Verification items for the finished model (mm, model axes). A direction names the side the tool comes from. Round coordinates to 2 decimals unless told otherwise and drop trailing zeros. Loops run counter-clockwise (first coordinate to the right, second up) from the corner with the lowest first, then second, coordinate; pieces in that order, holes last. Notation, with made-up numbers: M 27.25,88.5 L 39.25,88.5 A28 cw 39.25,115.5 Z; hole C 56,-10 d9. An arc over 180 degrees is marked long. Write item = value, one per line. Start each with the question number.
from build123d import *

# Parameters (mm, degrees)
EXTRUDE_THIN1_DEPTH = 34.154055886
SKETCH5_R           = 1.15
SKETCH5_W           = 12.978284002
SKETCH5_H           = 24
CUT_EXTRUDE7_DEPTH  = 8
SKETCH6_W           = 17.6
SKETCH6_H           = 13.993236592
SKETCH6_H_2         = 12.157086016
CUT_EXTRUDE8_DEPTH  = 29
SKETCH7_R           = 1.45
CUT_EXTRUDE9_DEPTH  = 33
SKETCH8_W           = 25.782103653
SKETCH8_H           = 13.229301
CUT_EXTRUDE10_DEPTH = 16


with BuildPart() as part:
    # Sketch1 → Extrude-Thin1 (new body)
    with BuildSketch(Plane.XY):
        Polygon((17.6, 0), (0, 0), (0, -20.0603024), (17.6, -20.0603024), (17.6, -23.662253526), (-3.601951126, -23.662253526), (-3.601951126, 3.601951126), (17.6, 3.601951126), align=None)
    extrude(amount=-EXTRUDE_THIN1_DEPTH)

    # Sketch5 → Cut-Extrude7 (cut)
    with BuildSketch(Plane(origin=(0, 0, 0), x_dir=(1, 0, 0), z_dir=(0, 1, 0))):
        with Locations(Location((7.452972893, 31.077545708, 0), (0, 0, 270))):
            Circle(SKETCH5_R)
        with Locations(Location((7.452972893, 3.870616702, 0), (0, 0, 270))):
            Circle(SKETCH5_R)
        with Locations((8.587190875, 17.5)):
            Rectangle(SKETCH5_W, SKETCH5_H)
    extrude(amount=CUT_EXTRUDE7_DEPTH, mode=Mode.SUBTRACT)

    # Sketch6 → Cut-Extrude8 (cut)
    with BuildSketch(Plane(origin=(0, 0, 0), x_dir=(1, 0, 0), z_dir=(0, 1, 0))):
        with Locations((8.8, 27.15743759)):
            Rectangle(SKETCH6_W, SKETCH6_H)
        with Locations((8.8, 6.078543008)):
            Rectangle(SKETCH6_W, SKETCH6_H_2)
    extrude(amount=-CUT_EXTRUDE8_DEPTH, mode=Mode.SUBTRACT)

    # Sketch7 → Cut-Extrude9 (cut)
    with BuildSketch(Plane(origin=(0, 0, 0), x_dir=(1, 0, 0), z_dir=(0, 1, 0))):
        with Locations(Location((4.880389158, 16.394356575, 0), (0, 0, 90))):
            Circle(SKETCH7_R)
        with Locations(Location((12.319153027, 16.394356575, 0), (0, 0, 90))):
            Circle(SKETCH7_R)
    extrude(amount=-CUT_EXTRUDE9_DEPTH, mode=Mode.SUBTRACT)

    # Sketch8 → Cut-Extrude10 (cut)
    with BuildSketch(Plane(origin=(0, 0, 0), x_dir=(0, 0, -1), z_dir=(1, 0, 0))):
        with Locations((16.964278219, -9.823443372)):
            Rectangle(SKETCH8_W, SKETCH8_H)
    extrude(amount=-CUT_EXTRUDE10_DEPTH, mode=Mode.SUBTRACT)


solid = part.part
1. Section check A-A, the plane z = -6. Enter the section's corners in (x, y), and give its area (3 significant figures).
2. Section check D-D, the plane x = 4.25. Enter the section's corners in (y, z).
3. Mould release check, pull along Y, two halves, no side actions. Record for faces 1 (the flat face through (3, -23.662, -16)), 2 (the flat face through (-2, -10, -29.855)), 3 (the flat face through (0, 3.602, -13)), 4 (the flat face through (9, -22, -20.161)): pulls with the +Y half, pulls with the -Y half, needs draft (parallel to the pull), parting line crosses it, or undercut.
4. Thickness scan on line 1 (Y direction, x = 15.75, z = -13); line 2 (Z direction, x = 5, y = -20.75); line 3 (X direction, y = -20.75, z = -28.5). Record the ranges inside material, lowest first.
5. Tool access check on faces 5 (the flat face through (-2, -3.209, -17)), 6 (the flat face through (9, -22, -12.157)), 7 (the flat face through (15.076, 2, -17)). Record the directions out of +Z, -Z, +X, -X, +Y, -Y that give a thin tool (end or side, any length) a straight path to the whole face; none if there is none.
6. Gauge pin test, flat ends, axial feed: P1, Ø3, axis at x = 7.5, z = -29.5, coming from the -Y side; P2, Ø3, axis at x = 4, z = -13, coming from the +Y side; P3, Ø6, axis at y = -12, z = -20, coming from the -X side; P4, Ø1.1, axis at x = 10.5, y = -22, coming from the -Z side. Record the tip position at first contact, or that the pin passes through.
7. Section check C-C, the plane x = 10. Enter the section's corners in (y, z), and give its area (3 significant figures).
8. Section check B-B, the plane y = -8. Enter the section's corners in (x, z), and give its area (3 significant figures).
Computed values:
q1.outline = M -3.6,-23.66 L 0,-23.66 L 0,-16.44 L -3.6,-16.44 Z; M -3.6,-3.21 L 0,-3.21 L 0,0 L 2.1,0 L 2.1,3.6 L -3.6,3.6 Z; M 15.08,0 L 17.6,0 L 17.6,3.6 L 15.08,3.6 Z
q1.area = 67.2 mm2
q2.outline = M -23.66,-20.16 L -20.06,-20.16 L -20.06,-17.7 L -23.66,-17.7 Z; M -23.66,-15.09 L -20.06,-15.09 L -20.06,-12.16 L -23.66,-12.16 Z; M 0,-34.15 L 3.6,-34.15 L 3.6,-29.5 L 0,-29.5 Z; M 0,-5.5 L 3.6,-5.5 L 3.6,0 L 0,0 Z
q3.face_1 = pulls with the -Y half
q3.face_2 = undercut
q3.face_3 = pulls with the +Y half
q3.face_4 = needs draft
q4.line_1 = -23.66 to -20.06, 0 to 3.6
q4.line_2 = -20.16 to -17.84, -14.95 to -12.16
q4.line_3 = -3.6 to 0
q5.face_5 = +X, -X
q5.face_6 = +Z, +X, -Y
q5.face_7 = +Y
q6.P1 = 0
q6.P2 = -20.06
q6.P3 = through
q6.P4 = -20.16
q7.outline = M -23.66,-20.16 L -20.06,-20.16 L -20.06,-12.16 L -23.66,-12.16 Z; M 0,-34.15 L 3.6,-34.15 L 3.6,-29.5 L 0,-29.5 Z; M 0,-5.5 L 3.6,-5.5 L 3.6,0 L 0,0 Z
q7.area = 65.4 mm2
q8.outline = M -3.6,-34.15 L 0,-34.15 L 0,-29.86 L -3.6,-29.86 Z; M -3.6,-4.07 L 0,-4.07 L 0,0 L -3.6,0 Z
q8.area = 30.2 mm2
